```python
from build123d import *

# Parameters (mm, degrees)
F1_DEPTH = 3.175
F2_R     = 2.54
F3_DEPTH = 12.7
F4_R     = 1.1938
F5_DEPTH = 2.54


with BuildPart() as f1:
    # F0 (on Front) → F1 (new body)
    with BuildSketch(Plane.XZ):
        with BuildLine():
            Line((41.275, 3.175), (3.175, 3.175))
            ThreePointArc((3.175, 3.175), (0, 0), (3.175, -3.175))
            Line((3.175, -3.175), (41.275, -3.175))
            ThreePointArc((41.275, -3.175), (44.45, 0), (41.275, 3.175))
        make_face()
    extrude(amount=F1_DEPTH)

    # F2 (on face) → F3 (join)
    with BuildSketch(Plane.XZ.offset(3.175)):
        with Locations((4.8514, 0)):
            Circle(F2_R)
    extrude(amount=F3_DEPTH)

    # F4 (on face) → F5 (join)
    with BuildSketch(Plane(origin=(0, 0, 0), x_dir=(-1, 0, 0), z_dir=(0, 1, 0))):
        with Locations((-16.51, 0)):
            Circle(F4_R)
        with Locations((-33.02, 0)):
            Circle(F4_R)
    extrude(amount=F5_DEPTH)


solid = f1.part
```
Model file for the job. Use its own axes, mm. A direction names the side the tool comes from. Give positions to 0.01 mm unless a question says otherwise; leave off trailing zeros. Loops run counter-clockwise (first coordinate to the right, second up) from the corner with the lowest first, then second, coordinate; pieces in that order, holes last. Notation, with made-up numbers: (-32.5, 76) -> (-8.5, 76) arc R25 cw to (-8.5, 95) -> close; hole circle Ø11 at (-17, 88.25). An arc over 180 degrees is marked (long way). Write each question's results on one line, items separated by ' | '.
(1) Probe line 1 along Y through (x, z) = (23, -0.5) (3 decimals); line 2 along Z through (x, y) = (5, -10); line 3 along Y through (x, z) = (17, 1) (3 decimals). List the from-to ranges inside material, lowest first.
Geometry results:
line 1: y = -3.175 to 0 | line 2: z = -2.54 to 2.54 | line 3: y = -3.175 to 2.54
(2) Pull direction X, two halves, no side cores. Call faces 3 (the cylindrical face through (34.213, 1.252, 0.052)), 4 (the flat face through (22, -2, 3.175)), 5 (the cylindrical face through (44.45, -1.57, -0.07)), 6 (the cylindrical face through (7.274, -9.436, 0.763)): released by +X, released by -X, zero draft, split by the parting line, or undercut.
Geometry results:
face 3: undercut | face 4: zero draft | face 5: released by +X | face 6: split by the parting line
(3) Cut at D-D on x = 5.5. List the corners of the cut face in (y, z) (3 decimals).
Geometry results:
outline: (-15.875, -2.456) -> (-3.175, -2.456) -> (-3.175, -3.175) -> (0, -3.175) -> (0, 3.175) -> (-3.175, 3.175) -> (-3.175, 2.456) -> (-15.875, 2.456) -> close
(4) Cut at A-A on x = 33.02. List the corners of the cut face in (y, z) (3 decimals).
Geometry results:
outline: (-3.175, -3.175) -> (0, -3.175) -> (0, -1.194) -> (2.54, -1.194) -> (2.54, 1.194) -> (0, 1.194) -> (0, 3.175) -> (-3.175, 3.175) -> close
(5) Flat gauge pins, fed straight in: pin 1 Ø5 at (x, y) = (19.5, -6.5) entering from -Z; pin 2 Ø3 at (y, z) = (-13.5, 0) entering from +X. Where does each tip first touch, or does it go through?
Geometry results:
pin 1: passes through | pin 2: stops at x = 7.39
(6) Tool access for faces 1 (the flat face through (22, -2, -3.175)), 2 (the cylindrical face through (17.39, 1.252, 0.807)): list every direction of +Z, -Z, +X, -X, +Y, -Y with a clear straight run to the whole face (end or side of a thin tool).
Geometry results:
face 1: -Z, +X, -X, +Y, -Y | face 2: +Y
(7) Cut at C-C on y = -11.5. List the corners of the cut face in (x, z).
Geometry results:
outline: circle Ø5.08 at (4.85, 0)
(8) Cut at B-B on z = 0. List the corners of the cut face in (x, y) (3 decimals).
Geometry results:
outline: (0, -3.175) -> (2.311, -3.175) -> (2.311, -15.875) -> (7.391, -15.875) -> (7.391, -3.175) -> (44.45, -3.175) -> (44.45, 0) -> (34.214, 0) -> (34.214, 2.54) -> (31.826, 2.54) -> (31.826, 0) -> (17.704, 0) -> (17.704, 2.54) -> (15.316, 2.54) -> (15.316, 0) -> (0, 0) -> close
